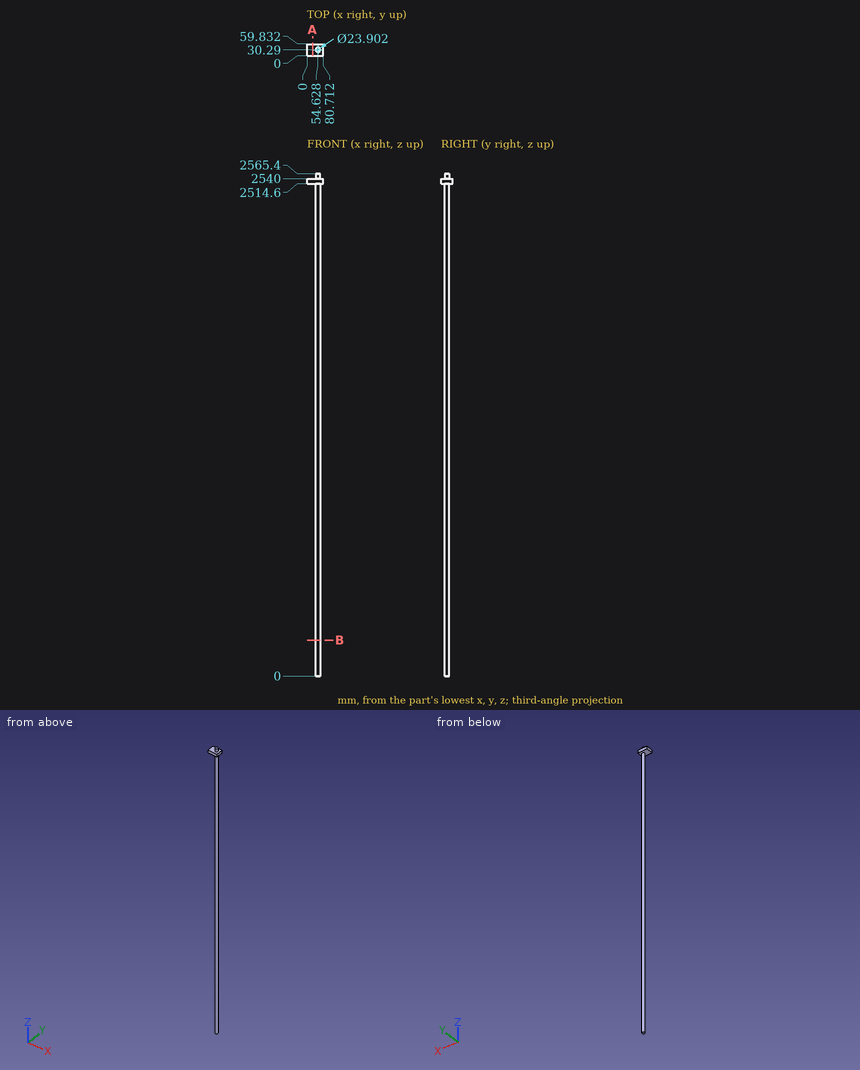
Design review of the part shown in the three views and the two pictorial views. Dimensions are in mm from the part's minimum x, y and z. Round coordinates to 2 decimals unless told otherwise and drop trailing zeros. Loops run counter-clockwise (first coordinate to the right, second up) from the corner with the lowest first, then second, coordinate; pieces in that order, holes last.
(1) Wall thickness on line 1 along Z through (x, y) = (47, 14); line 2 along X through (y, z) = (27.5, 2018); line 3 along X through (y, z) = (29.5, 900): over which ranges is each line inside the solid? List them lowest first.
Returned:
line 1: z = 2514.6 to 2540
line 2: x = 43.01 to 66.25
line 3: x = 42.7 to 66.55
(2) We need section B-B (z = 183). Give the boundary of the cut face in (x, y).
Returned:
outline: circle Ø23.9 at (54.63, 30.29)
(3) We need section A-A (x = 27.5). Give the boundary of the cut face in (y, z), plus the area to 3 significant figures.
Returned:
outline: (0, 2514.6) - (59.83, 2514.6) - (59.83, 2540) - (0, 2540) - close
area: 1,520 mm2
(4) Clearance check with flat-ended pins moving along their axes: P1, Ø5, axis at y = 19, z = 2235.5, coming from the +X side (1 decimal); P2, Ø2, axis at x = 48.5, z = 2190, coming from the -Y side (1 decimal); P3, Ø12, axis at y = 47, z = 1625, coming from the +X side (1 decimal). State where each tip first meets the part, or that it passes through.
Returned:
P1: stops at x = 62.7
P2: stops at y = 19.5
P3: stops at x = 59.9
